Input: dimensioned drawing with shaded views. Units: mm. Origin: part minimum x, y, z. A direction names the side the tool comes from. Coordinates: 2 decimals unless noted, no trailing zeros. Loops run counter-clockwise (first coordinate to the right, second up) from the corner with the lowest first, then second, coordinate; pieces in that order, holes last. Notation, with made-up numbers: (-26, 10.25) -> (-21, 10.25) arc R29 ccw to (-21, 34.25) -> close; hole circle Ø2 at (78, 16.25). An arc over 180 degrees is marked (long way). Answer as CSV lines item,"result".
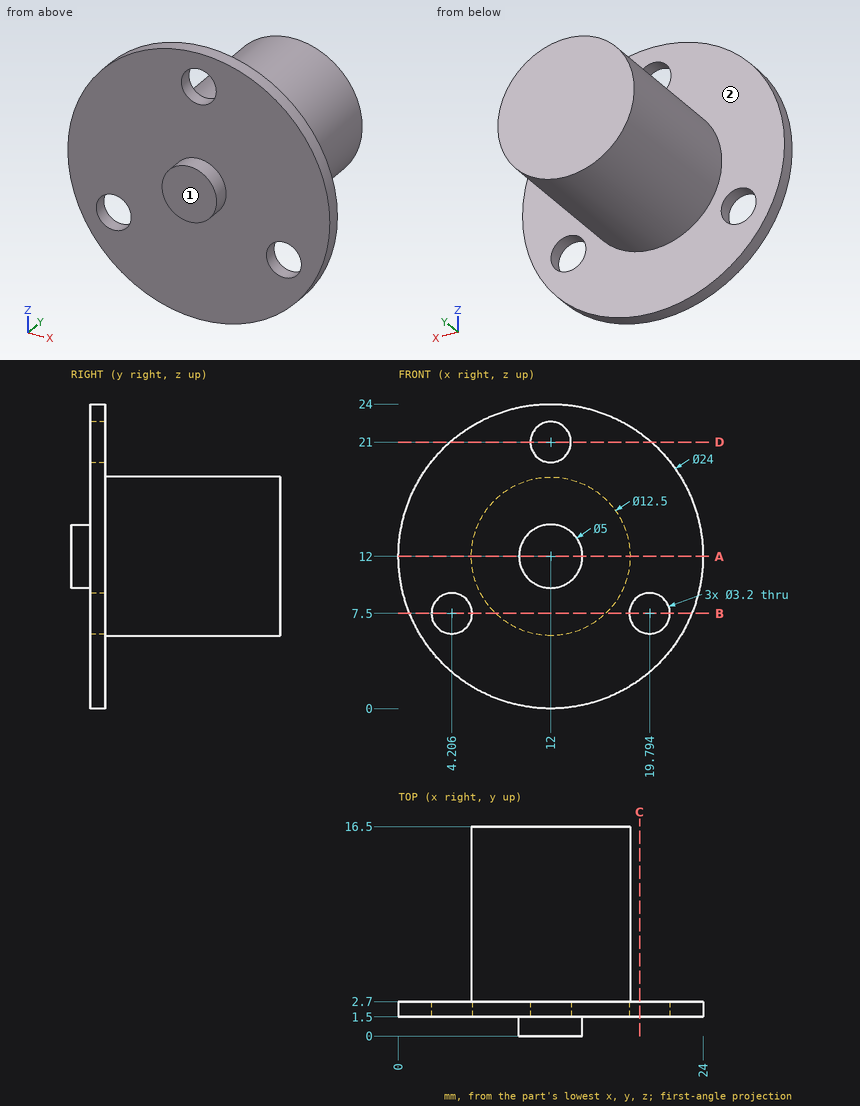
(1) Access query for the marked faces 1 and 2. Directions: +Z, -Z, +X, -X, +Y, -Y. A direction counts if a zero-diameter tool reaches every point of the face in a straight line with its end or side. Return the directions, or none.
Computed values:
face 1,"+Z, -Z, +X, -X, -Y"
face 2,"+Y"
(2) Cut plane C-C (x = 19). Return the cut outline in (y, z).
Computed values:
outline,"(1.5, 2.25) -> (2.7, 2.25) -> (2.7, 6.11) -> (1.5, 6.11) -> close; (1.5, 8.89) -> (2.7, 8.89) -> (2.7, 21.75) -> (1.5, 21.75) -> close"
(3) Pin query (flat end, axial travel): pin 1 Ø5 at (x, z) = (19.79, 7.5) entering from -Y; pin 2 Ø1.5 at (x, y) = (9.5, 12) entering from -Z; pin 3 Ø3.5 at (x, z) = (12, 21) entering from +Y. Return the tip coordinate at first contact, or that it passes through.
Computed values:
pin 1,"y = 1.5"
pin 2,"z = 6"
pin 3,"y = 2.7"
(4) Material intervals for L1, parallel to Y at x = 21.25, z = 10.75; L2, parallel to Y at x = 15, z = 9.5; L3, parallel to X at y = 2.45, z = 21, sorted ascending. Write a range as [from, to].
Computed values:
L1,"[1.5, 2.7]"
L2,"[1.5, 16.5]"
L3,"[4.06, 10.4], [13.6, 19.94]"
(5) Cut plane D-D (z = 21). Return the cut outline in (x, y), then the cut area to 3 significant figures.
Computed values:
outline,"(4.06, 1.5) -> (10.4, 1.5) -> (10.4, 2.7) -> (4.06, 2.7) -> close; (13.6, 1.5) -> (19.94, 1.5) -> (19.94, 2.7) -> (13.6, 2.7) -> close"
area,"15.2 mm^2"
(6) Cut plane B-B (z = 7.5). Return the cut outline in (x, y), then the cut area to 3 significant figures.
Computed values:
outline,"(0.88, 1.5) -> (2.61, 1.5) -> (2.61, 2.7) -> (0.88, 2.7) -> close; (5.81, 1.5) -> (18.19, 1.5) -> (18.19, 2.7) -> (16.34, 2.7) -> (16.34, 16.5) -> (7.66, 16.5) -> (7.66, 2.7) -> (5.81, 2.7) -> close; (21.39, 1.5) -> (23.12, 1.5) -> (23.12, 2.7) -> (21.39, 2.7) -> close"
area,"139 mm^2"
(7) Cut plane A-A (z = 12). Return the cut outline in (x, y), then the cut area to 3 significant figures.
Computed values:
outline,"(0, 1.5) -> (9.5, 1.5) -> (9.5, 0) -> (14.5, 0) -> (14.5, 1.5) -> (24, 1.5) -> (24, 2.7) -> (18.25, 2.7) -> (18.25, 16.5) -> (5.75, 16.5) -> (5.75, 2.7) -> (0, 2.7) -> close"
area,"209 mm^2"
